Read the model definition and answer for the solid it produces. Units are mm, in the model's axes. Coordinates: 2 decimals unless noted, no trailing zeros. Loops run counter-clockwise (first coordinate to the right, second up) from the corner with the lowest first, then second, coordinate; pieces in that order, holes last.
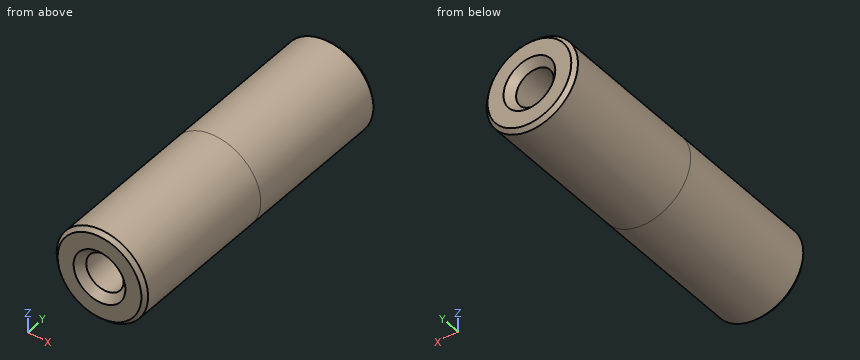
Autodesk Inventor part; units mm, degrees
ref_plane "YZ Plane" through (0, 0, 0) normal (1, 0, 0) x (0, 1, 0)
ref_plane "XZ Plane" through (0, 0, 0) normal (0, 1, 0) x (-1, 0, 0)
ref_plane "XY Plane" through (0, 0, 0) normal (0, 0, 1) x (1, 0, 0)
sketch "スケッチ1" plane through (0, 0, 0) normal (0, 1, 0) x (-1, 0, 0)
  circle A0 centre (0, 0) radius 3
  dimension "d0" = 6
extrude "押し出し1" add sketch "スケッチ1" along normal mid plane 20
sketch "スケッチ2" plane through (0, 10, 0) normal (0, 1, 0) x (1, 0, 0)
  point P0 (0, 0)
  point P1 (0, 0)
hole "穴1" at (0, 10, 0) direction (0, -1, 0) diameter 2.459 depth 10 countersink diameter 3.4 countersink angle 90
sketch "スケッチ3" plane through (0, -10, 0) normal (0, -1, 0) x (1, 0, 0)
  point P0 (0, 0)
  point P1 (0, 0)
hole "穴2" at (0, -10, 0) direction (0, 1, 0) diameter 2.459 depth 10 countersink diameter 3.4 countersink angle 90
chamfer "面取り1" distance 0.25 angle 45 2 edges at (3, -10, 0) (3, 10, 0)
properties part number "Spacer_M3D6L60" material "アルミニウム 6061"
Q1. Straight lines are drawn through the part: probe 1 along Z at (x, y) = (0, 6); probe 2 along Z at (x, y) = (0.5, -4.25). For each, find the intervals that lie inside material, in ascending order.
Findings below:
probe 1: z = -3 to -1.23, 1.23 to 3
probe 2: z = -2.96 to -1.12, 1.12 to 2.96
Q2. A cutting plane is placed at C-C (y = -5.75). Give the vertices of the cut face in (x, z), then the cut area to 3 significant figures.
Findings below:
outline: circle Ø6 at (0, 0); hole circle Ø2.46 at (0, 0)
area: 23.5 mm2
Q3. Flat-ended cylindrical pins translate along their axes: pin 1 Ø1.5 at (x, y) = (2, -6.5) entering from +Z; pin 2 Ø1 at (x, z) = (-1, 0.5) entering from +Y; pin 3 Ø2 at (y, z) = (0.5, 2) entering from +X; pin 4 Ø2 at (x, z) = (0, 0) entering from -Y. Find the tip coordinate at first contact, or state that the pin passes through.
Findings below:
pin 1: stops at z = 2.73
pin 2: stops at y = 9.92
pin 3: stops at x = 2.83
pin 4: passes through
Q4. A cutting plane is placed at B-B (x = 0). Give the vertices of the cut face in (y, z).
Findings below:
outline: (-10, -2.75) - (-9.75, -3) - (9.75, -3) - (10, -2.75) - (10, -1.7) - (9.53, -1.23) - (-9.53, -1.23) - (-10, -1.7) - close; (-10, 1.7) - (-9.53, 1.23) - (9.53, 1.23) - (10, 1.7) - (10, 2.75) - (9.75, 3) - (-9.75, 3) - (-10, 2.75) - close
Q5. A cutting plane is placed at A-A (z = 0). Give the vertices of the cut face in (x, y), then the cut area to 3 significant figures.
Findings below:
outline: (-3, -9.75) - (-2.75, -10) - (-1.7, -10) - (-1.23, -9.53) - (-1.23, 9.53) - (-1.7, 10) - (-2.75, 10) - (-3, 9.75) - close; (1.23, -9.53) - (1.7, -10) - (2.75, -10) - (3, -9.75) - (3, 9.75) - (2.75, 10) - (1.7, 10) - (1.23, 9.53) - close
area: 70.3 mm2
